Part model, mm, in its own coordinate system. A direction names the side the tool comes from. Give positions to 0.01 mm unless a question says otherwise; leave off trailing zeros. Write each loop counter-clockwise with the first axis right and the second up, starting at its lowest first coordinate (ties: lowest second). Pieces come first, ordered by that corner, then holes. Notation, with made-up numbers: M -19.5,5.25 L -0.5,5.25 A17 ccw -0.5,29.25 Z; hole C -3,-10.5 d10. An arc over 180 degrees is marked long. Use CSV: the item, a comma, the result in double quotes. Start each with the question number.
1. Band-saw the part on B-B, the plane x = 23. List the corners of the cut face in (y, z) (1 decimal), then the cut area to 3 significant figures.
2. Drill centre lines: line 1 along Y through (x, z) = (12, 0); line 2 along Y through (x, z) = (21.5, 5); line 3 along X through (y, z) = (18, 2.5). Where is each one in solid material? Low to high. Write a range as from..to.
3. Band-saw the part on A-A, the plane x = 12. List the corners of the cut face in (y, z) (1 decimal).
4. Drop flat-ended pins along their axis: pin 1 Ø4 at (x, z) = (32, -14.5) entering from -Y; pin 2 Ø5 at (x, y) = (41.5, 7.5) entering from +Z; pin 3 Ø8 at (x, y) = (30, 8.5) entering from -Z. Give the stop position or say it passes through.
5. 3-axis set-ups, long thin cutter, end or side, ignore diameter. For faces 1 (the face through (0.184, -9.511, -16.382)), 2 (the face through (22.26, 17.48, -3.88)): which of +Z, -Z, +X, -X, +Y, -Y reach the whole face in a straight line?
6. Mould opens along Z. For faces 3 (the face through (18.3, -7.5, -8.2)), 4 (the face through (40.663, 1.732, -0.385)), 5 (the face through (0.184, -18.943, 0.046)), 6 (the face through (20.394, -9.505, -16.37)) say: pulls with the +Z half, pulls with the -Z half, needs draft (parallel to the pull), parting line crosses it, or undercut.
from build123d import *

# Parameters (mm, degrees)
BASENUT_DEPTH = 20.574


with BuildPart() as part:
    # BaseNutSke → BaseNut (new body)
    with BuildSketch(Plane(origin=(0, 0, 0), x_dir=(0, 0, -1), z_dir=(1, 0, 0))):
        Polygon((18.25625, 10.540250852), (18.25625, -10.540250852), (0, -21.080501704), (-18.25625, -10.540250852), (-18.25625, 10.540250852), (0, 21.080501704), align=None)
    extrude(amount=BASENUT_DEPTH)

    # Sketch3 → Crown (revolve)
    with BuildSketch(Plane.XY, mode=Mode.PRIVATE) as crown_sk:
        with BuildLine():
            Line((50.038, 0), (0, 0))
            Line((0, 0), (0, 17.907))
            Line((0, 17.907), (23.89386723, 17.907))
            ThreePointArc((23.89386723, 17.907), (38.686643155, 13.843242093), (49.327308282, 2.792604396))
            ThreePointArc((49.327308282, 2.792604396), (49.857539852, 1.440808977), (50.038, 0))
        make_face()
    revolve(crown_sk.sketch.rotate(Axis((0, 0, 0), (1, 0, 0)), 90), axis=Axis((0, 0, 0), (1, 0, 0)))

    # Sketch4 → DoubleChamfer (revolve, cut)
    with BuildSketch(Plane.XY, mode=Mode.PRIVATE) as doublechamfer_sk:
        Polygon((0, 18.25625), (1.949893068, 25.53335), (18.624460993, 25.53335), (20.574, 18.25625), (33.274, 18.25625), (33.274, 43.65625), (-12.7, 43.65625), (-12.7, 18.25625), align=None)
    revolve(doublechamfer_sk.sketch.rotate(Axis((0, 0, 0), (1, 0, 0)), 90), axis=Axis((0, 0, 0), (1, 0, 0)), mode=Mode.SUBTRACT)

    # Sketch5 → TapDrill (revolve, cut)
    with BuildSketch(Plane.XY, mode=Mode.PRIVATE) as tapdrill_sk:
        Polygon((0, 11.1125), (35.052, 11.1125), (41.729063629, 0), (0, 0), align=None)
    revolve(tapdrill_sk.sketch.rotate(Axis((0, 0, 0), (1, 0, 0)), 90), axis=Axis((0, 0, 0), (1, 0, 0)), mode=Mode.SUBTRACT)

    # EndChamferSketch → EndChamfer (revolve, cut)
    with BuildSketch(Plane.XY, mode=Mode.PRIVATE) as endchamfer_sk:
        Polygon((-0.0254, 12.7), (0.0254, 12.7), (1.248137414, 10.95375), (-0.0254, 10.95375), align=None)
    revolve(endchamfer_sk.sketch.rotate(Axis((-3.175, 0, 0), (-1, 0, 0)), 270), axis=Axis((-3.175, 0, 0), (-1, 0, 0)), mode=Mode.SUBTRACT)


solid = part.part
Output:
1,outline,"C 0,0 d35.8; hole C 0,0 d22.2"
1,area,"619 mm²"
2,line 1,"y = -21.08..-11.11, 11.11..21.08"
2,line 2,"y = -17.19..-9.92, 9.92..17.19"
2,line 3,"x = 0..20.57"
3,outline,"M -21.1,0 L -10.5,-18.3 L 10.5,-18.3 L 21.1,0 L 10.5,18.3 L -10.5,18.3 Z; hole C 0,0 d22.2"
4,pin 1,"stops at y = -11.3"
4,pin 2,"stops at z = 11.92"
4,pin 3,"stops at z = -16.88"
5,face 1,"-Z, -X, -Y"
5,face 2,"+X"
6,face 3,"undercut"
6,face 4,"undercut"
6,face 5,"parting line crosses it"
6,face 6,"pulls with the -Z half"
